from build123d import *

# Parameters (mm, degrees)
SKETCH1_W           = 62.3
SKETCH1_H           = 39.5
SKETCH1_R           = 12.5
SKETCH1_R_2         = 2.55
BOSS_EXTRUDE1_DEPTH = 3
FILLET1_R           = 5


with BuildPart() as part:
    # Sketch1 → Boss-Extrude1 (new body)
    with BuildSketch(Plane.XY):
        with Locations((31.15, 19.75)):
            Rectangle(SKETCH1_W, SKETCH1_H)
        with Locations((19.75, 19.75)):
            Circle(SKETCH1_R, mode=Mode.SUBTRACT)
        with Locations((52.3, 29.75)):
            Circle(SKETCH1_R_2, mode=Mode.SUBTRACT)
        with Locations((52.3, 9.75)):
            Circle(SKETCH1_R_2, mode=Mode.SUBTRACT)
        with BuildLine():
            Line((5.346015511, 36.346015511), (7.846015511, 33.846015511))
            ThreePointArc((7.846015511, 33.846015511), (7.846015511, 31.653984489), (5.653984489, 31.653984489))
            Line((5.653984489, 31.653984489), (3.153984489, 34.153984489))
            ThreePointArc((3.153984489, 34.153984489), (3.153984489, 36.346015511), (5.346015511, 36.346015511))
        make_face(mode=Mode.SUBTRACT)
        with BuildLine():
            Line((34.153984489, 36.346015511), (31.653984489, 33.846015511))
            ThreePointArc((31.653984489, 33.846015511), (31.653984489, 31.653984489), (33.846015511, 31.653984489))
            Line((33.846015511, 31.653984489), (36.346015511, 34.153984489))
            ThreePointArc((36.346015511, 34.153984489), (36.346015511, 36.346015511), (34.153984489, 36.346015511))
        make_face(mode=Mode.SUBTRACT)
        with BuildLine():
            Line((34.153984489, 3.153984489), (31.653984489, 5.653984489))
            ThreePointArc((31.653984489, 5.653984489), (31.653984489, 7.846015511), (33.846015511, 7.846015511))
            Line((33.846015511, 7.846015511), (36.346015511, 5.346015511))
            ThreePointArc((36.346015511, 5.346015511), (36.346015511, 3.153984489), (34.153984489, 3.153984489))
        make_face(mode=Mode.SUBTRACT)
        with BuildLine():
            Line((5.346015511, 3.153984489), (7.846015511, 5.653984489))
            ThreePointArc((7.846015511, 5.653984489), (7.846015511, 7.846015511), (5.653984489, 7.846015511))
            Line((5.653984489, 7.846015511), (3.153984489, 5.346015511))
            ThreePointArc((3.153984489, 5.346015511), (3.153984489, 3.153984489), (5.346015511, 3.153984489))
        make_face(mode=Mode.SUBTRACT)
    extrude(amount=BOSS_EXTRUDE1_DEPTH)

    # Fillet1
    fillet1_edges = [part.edges().sort_by_distance(p)[0] for p in [
        (0, 39.5, 1.5),
        (62.3, 39.5, 1.5),
        (62.3, 0, 1.5),
        (0, 0, 1.5),
    ]]
    fillet(fillet1_edges, radius=FILLET1_R)


solid = part.part
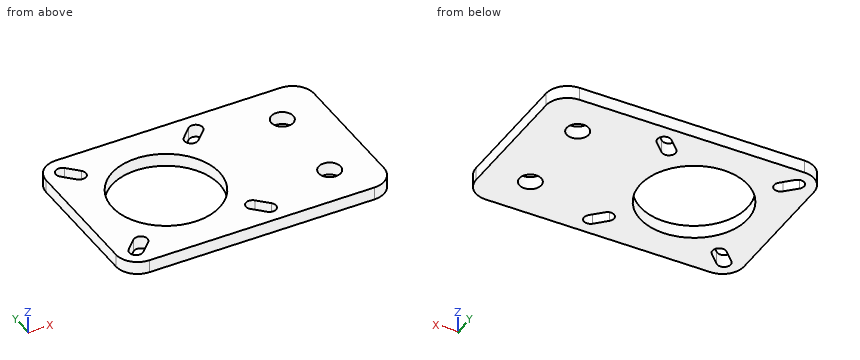
Verification items for the finished model (mm, model axes). Coordinates: 2 decimals unless noted, no trailing zeros. Loops run counter-clockwise (first coordinate to the right, second up) from the corner with the lowest first, then second, coordinate; pieces in that order, holes last. Notation, with made-up numbers: (17.25, 77) -> (45.25, 77) arc R9 ccw to (45.25, 88) -> close; hole circle Ø8 at (64.25, -24.75). An arc over 180 degrees is marked (long way). Answer as a JSON object with one key per item and string values. Group by question number.
Item 1: Sectioned sample at A-A on y = 9.75. Record the boundary of the cut face in (x, z), plus the area to 3 significant figures.
Item 2: Sectioned sample at C-C on y = 19.75. Record the boundary of the cut face in (x, z).
Item 3: Sectioned sample at D-D on z = 1.25. Record the boundary of the cut face in (x, y), plus the area to 3 significant figures.
Item 4: Sectioned sample at B-B on x = 19.75. Record the boundary of the cut face in (y, z).
Item 5: Scan lines: probe 1 along Y at (x, z) = (52.3, 0.6); probe 2 along X at (y, z) = (20, 1.65); probe 3 along Y at (x, z) = (19.75, 1.85). Record each from-to range of solid material in increasing order.
Evaluation:
{
 "1": {"outline": "(0, 0) -> (12.25, 0) -> (12.25, 3) -> (0, 3) -> close; (27.25, 0) -> (49.75, 0) -> (49.75, 3) -> (27.25, 3) -> close; (54.85, 0) -> (62.3, 0) -> (62.3, 3) -> (54.85, 3) -> close", "area": "127 mm²"},
 "2": {"outline": "(0, 0) -> (7.25, 0) -> (7.25, 3) -> (0, 3) -> close; (32.25, 0) -> (62.3, 0) -> (62.3, 3) -> (32.25, 3) -> close"},
 "3": {"outline": "(0, 5) arc R5 ccw to (5, 0) -> (57.3, 0) arc R5 ccw to (62.3, 5) -> (62.3, 34.5) arc R5 ccw to (57.3, 39.5) -> (5, 39.5) arc R5 ccw to (0, 34.5) -> close; hole (3.15, 5.35) arc R1.55 ccw to (5.35, 3.15) -> (7.85, 5.65) arc R1.55 ccw to (5.65, 7.85) -> close; hole (3.15, 34.15) -> (5.65, 31.65) arc R1.55 ccw to (7.85, 33.85) -> (5.35, 36.35) arc R1.55 ccw to start; hole circle Ø25 at (19.75, 19.75); hole (31.65, 5.65) -> (34.15, 3.15) arc R1.55 ccw to (36.35, 5.35) -> (33.85, 7.85) arc R1.55 ccw to start; hole (31.65, 33.85) arc R1.55 ccw to (33.85, 31.65) -> (36.35, 34.15) arc R1.55 ccw to (34.15, 36.35) -> close; hole circle Ø5.1 at (52.3, 9.75); hole circle Ø5.1 at (52.3, 29.75)", "area": "1,830 mm²"},
 "4": {"outline": "(0, 0) -> (7.25, 0) -> (7.25, 3) -> (0, 3) -> close; (32.25, 0) -> (39.5, 0) -> (39.5, 3) -> (32.25, 3) -> close"},
 "5": {"probe 1": "y = 0 to 7.2, 12.3 to 27.2, 32.3 to 39.5", "probe 2": "x = 0 to 7.25, 32.25 to 62.3", "probe 3": "y = 0 to 7.25, 32.25 to 39.5"}
}
